Verification items for the finished model (mm, model axes). A direction names the side the tool comes from. Coordinates: 2 decimals unless noted, no trailing zeros. Loops run counter-clockwise (first coordinate to the right, second up) from the corner with the lowest first, then second, coordinate; pieces in that order, holes last. Notation, with made-up numbers: (-8.5, 7) - (26.5, 7) arc R32 cw to (26.5, 38) - close; hole circle Ø11 at (-26.5, 72.5). An arc over 180 degrees is marked (long way). Answer as CSV lines item,"result". Start each with the question number.
1. Set-up check for faces 5 (the flat face through (56, 0, 3)), 6 (the cylindrical face through (1, 18, 78)): record each of +Z, -Z, +X, -X, +Y, -Y from which the full face is reachable in a straight line by a thin tool's end or side.
2. Gauge pin test, flat ends, axial feed: P1, Ø20, axis at x = 46, y = -8, coming from the +Z side; P2, Ø20, axis at y = 8, z = 48, coming from the +X side; P3, Ø8.5, axis at y = 0, z = 59, coming from the +X side. Record the tip position at first contact, or that the pin passes through.
3. Material ranges on line 1 (Z direction, x = 2.35, y = 0); line 2 (Z direction, x = 2.25, y = 0); line 3 (Z direction, x = 65, y = -10.5), recorded low to high. Write a range as [from, to].
4. Cross-section at C-C (z = 29). Enter the section's corners in (x, y), plus the area to 3 significant figures.
5. Cross-section at D-D (y = 8.5). Enter the section's corners in (x, z).
6. Release check for a two-part mould opening along X. For faces 1 (the cylindrical face through (67, 0, 2)), 2 (the cylindrical face through (1, -18, 78)), 3 (the flat face through (104, 0, 1)), 4 (the cylindrical face through (1.711, -0.28, 1.804)) record: pulls with the +X half, pulls with the -X half, needs draft (parallel to the pull), parting line crosses it, or undercut.
7. Cross-section at A-A (x = 34). Enter the section's corners in (y, z).
8. Cross-section at B-B (y = 0). Enter the section's corners in (x, z).
```python
from build123d import *

# Parameters (mm, degrees)
F1_DEPTH = 20
F2_R     = 5
F3_R     = 7
F4_DEPTH = 25
F5_R     = 7
F6_DEPTH = 25


with BuildPart() as f1:
    # F0 (on Front) → F1 (new body, symmetric)
    with BuildSketch(Plane.XZ):
        with BuildLine():
            Line((0, 79), (0, 6))
            ThreePointArc((0, 6), (1.757359, 1.757359), (6, 0))
            Line((6, 0), (104, 0))
            Line((104, 0), (104, 3))
            Line((104, 3), (7, 3))
            ThreePointArc((7, 3), (4.171573, 4.171573), (3, 7))
            Line((3, 7), (3, 79))
            Line((3, 79), (0, 79))
        make_face()
    extrude(amount=F1_DEPTH, both=True)

    # F2
    f2_edges = [f1.edges().sort_by_distance(p)[0] for p in [
        (1.5, -20, 79),
        (1.5, 20, 79),
        (104, 20, 1.5),
        (104, -20, 1.5),
    ]]
    fillet(f2_edges, radius=F2_R)

    # F3 (on face) → F4 (cut)
    with BuildSketch(Plane.XY.offset(3)):
        with Locations((34, 0)):
            Circle(F3_R)
        with Locations((74, 0)):
            Circle(F3_R)
    extrude(amount=-F4_DEPTH, mode=Mode.SUBTRACT)

    # F5 (on face) → F6 (cut)
    with BuildSketch(Plane.YZ.offset(3)):
        with Locations((0, 59)):
            Circle(F5_R)
        with Locations((0, 29)):
            Circle(F5_R)
    extrude(amount=-F6_DEPTH, mode=Mode.SUBTRACT)


solid = f1.part
```
Values follow:
1,face 5,"+Z, +X, +Y, -Y"
1,face 6,"+Z, +X, -X, +Y"
2,P1,"stops at z = 3"
2,P2,"stops at x = 3"
2,P3,"passes through"
3,line 1,"z = [1.24, 22], [36, 52], [66, 79]"
3,line 2,"z = [1.32, 22], [36, 52], [66, 79]"
3,line 3,"z = [0, 3]"
4,outline,"(0, -20) - (3, -20) - (3, -7) - (0, -7) - close; (0, 7) - (3, 7) - (3, 20) - (0, 20) - close"
4,area,"78.0 mm²"
5,outline,"(0, 6) arc R6 ccw to (6, 0) - (104, 0) - (104, 3) - (7, 3) arc R4 cw to (3, 7) - (3, 79) - (0, 79) - close"
6,face 1,"undercut"
6,face 2,"needs draft"
6,face 3,"pulls with the +X half"
6,face 4,"pulls with the -X half"
7,outline,"(-20, 0) - (-7, 0) - (-7, 3) - (-20, 3) - close; (7, 0) - (20, 0) - (20, 3) - (7, 3) - close"
8,outline,"(0, 6) arc R6 ccw to (6, 0) - (27, 0) - (27, 3) - (7, 3) arc R4 cw to (3, 7) - (3, 22) - (0, 22) - close; (0, 36) - (3, 36) - (3, 52) - (0, 52) - close; (0, 66) - (3, 66) - (3, 79) - (0, 79) - close; (41, 0) - (67, 0) - (67, 3) - (41, 3) - close; (81, 0) - (104, 0) - (104, 3) - (81, 3) - close"
